Here's the drawing with two shaded views (mm, measured from the low corner). I have some questions. A direction names the side the tool comes from. Give positions to 0.01 mm unless a question says otherwise; leave off trailing zeros. Write each loop counter-clockwise with the first axis right and the second up, starting at its lowest first coordinate (ties: lowest second). Pieces come first, ordered by that corner, then holes. Notation, with made-up numbers: (42.5, -22) -> (99.5, -22) arc R18 ccw to (99.5, -2) -> close; hole circle Ø2 at (60, 24.5). An arc over 180 degrees is marked (long way). One line per item, written item: value.
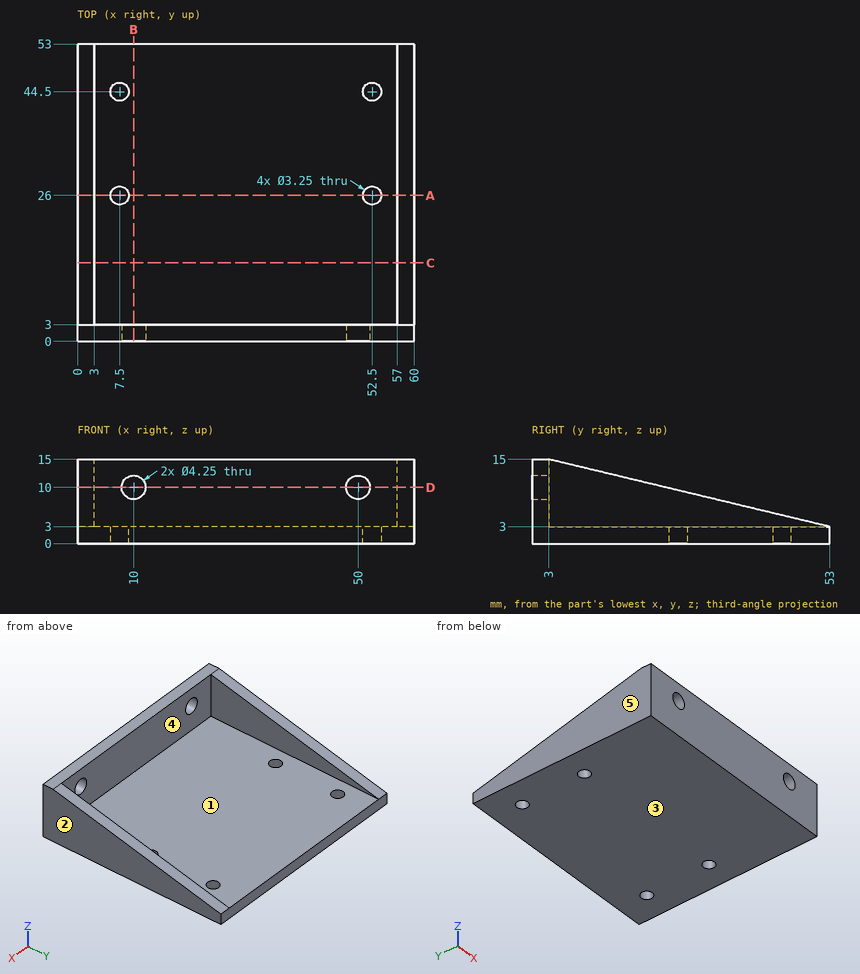
1) If we section it at D-D (z = 10): Write out the boundary of the cut face in (x, y) (3 decimals), and give its area (4 significant figures).
Answer list:
outline: (0, 0) -> (7.875, 0) -> (7.875, 3) -> (3, 3) -> (3, 23.833) -> (0, 23.833) -> close; (12.125, 0) -> (47.875, 0) -> (47.875, 3) -> (12.125, 3) -> close; (52.125, 0) -> (60, 0) -> (60, 23.833) -> (57, 23.833) -> (57, 3) -> (52.125, 3) -> close
area: 279.5 mm^2
2) I need wall thicknesses on L1, parallel to X at y = 1.1, z = 10 (3 decimals); L2, parallel to Y at x = 52.5, z = 2.15 (3 decimals); L3, parallel to X at y = 22, z = 3.75. Which ranges of each line are inside material? Lowest first, please.
Answer list:
L1: x = 0 to 7.875, 12.125 to 47.875, 52.125 to 60
L2: y = 0 to 24.375, 27.625 to 42.875, 46.125 to 53
L3: x = 0 to 3, 57 to 60
3) If we section it at A-A (y = 26): Write out the boundary of the cut face in (x, z) (3 decimals).
Answer list:
outline: (0, 0) -> (5.875, 0) -> (5.875, 3) -> (3, 3) -> (3, 9.48) -> (0, 9.48) -> close; (9.125, 0) -> (50.875, 0) -> (50.875, 3) -> (9.125, 3) -> close; (54.125, 0) -> (60, 0) -> (60, 9.48) -> (57, 9.48) -> (57, 3) -> (54.125, 3) -> close
4) If we section it at B-B (x = 10): Write out the boundary of the cut face in (y, z) (3 decimals).
Answer list:
outline: (0, 0) -> (53, 0) -> (53, 3) -> (3, 3) -> (3, 7.875) -> (0, 7.875) -> close; (0, 12.125) -> (3, 12.125) -> (3, 15) -> (0, 15) -> close
5) Will these pins go through, and if not, where does the flat tip stop? pin 1 (5.5 mm diameter, centred on x = 10, z = 10, fed in from +Y); pin 2 (3.5 mm diameter, centred on x = 7.5, y = 44.5, fed in from -Z); pin 3 (6 mm diameter, centred on x = 14, y = 9.5, fed in from +Z).
Answer list:
pin 1: stops at y = 3
pin 2: stops at z = 0
pin 3: stops at z = 3
6) For the marked faces 1 and 2, which set-ups out of +Z, -Z, +X, -X, +Y, -Y let a thin tool reach every point of the face, with its end or its side?
Answer list:
face 1: +Z, +Y
face 2: +Z, -Z, +X, +Y, -Y
7) If we section it at C-C (y = 14): Write out the boundary of the cut face in (x, z).
Answer list:
outline: (0, 0) -> (60, 0) -> (60, 12.36) -> (57, 12.36) -> (57, 3) -> (3, 3) -> (3, 12.36) -> (0, 12.36) -> close
8) We'd pull the mould along X, two halves only. Please class the marked faces 3, 4 and 5: released by +X, released by -X, zero draft, split by the parting line, or undercut.
Answer list:
face 3: zero draft
face 4: undercut
face 5: released by -X
